Geometry check sheet. Reference: drawing and pictorial views, mm from the part's lowest x, y, z. A direction names the side the tool comes from. Round coordinates to 2 decimals unless told otherwise and drop trailing zeros. Write each loop counter-clockwise with the first axis right and the second up, starting at its lowest first coordinate (ties: lowest second). Pieces come first, ordered by that corner, then holes. Notation, with made-up numbers: (29.5, -8) -> (60.5, -8) arc R30 cw to (60.5, 26) -> close; hole circle Ø1 at (84, 34.5). An arc over 180 degrees is marked (long way). Write item = value, one per line.
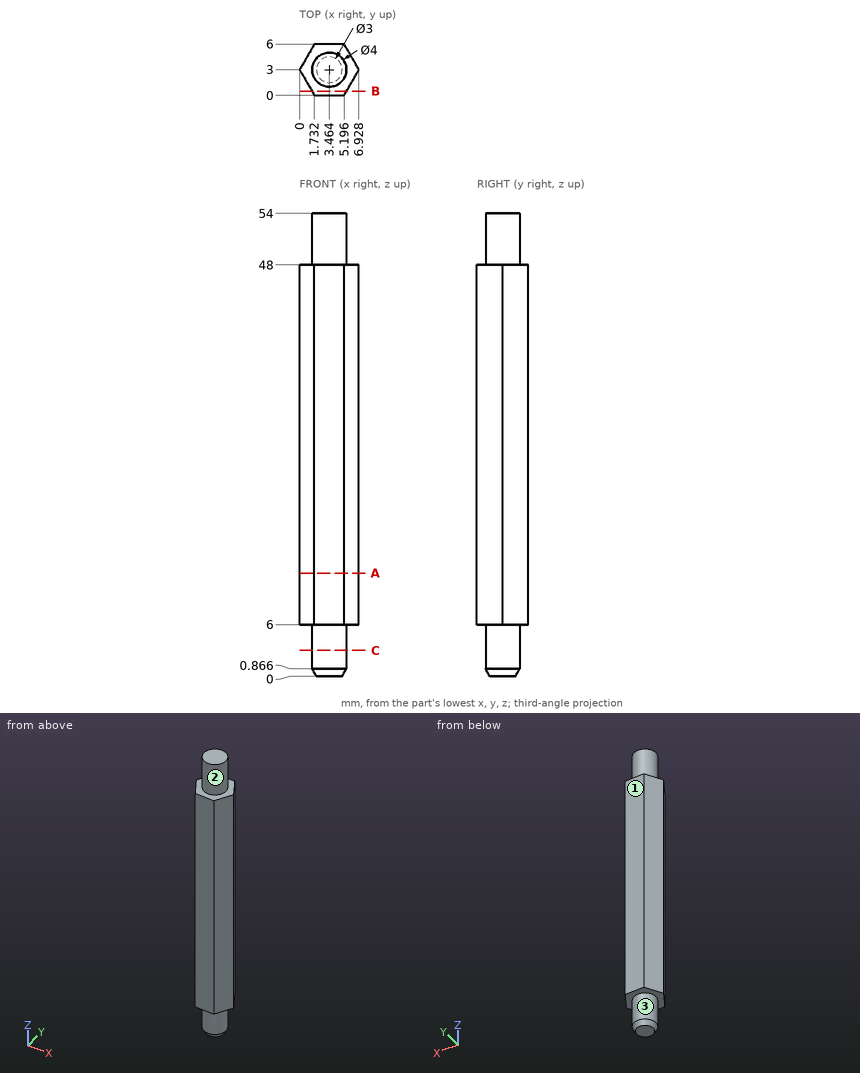
(1) Access from +Z, -Z, +X, -X, +Y, -Y to the whole of each face (thin tool, end or side, straight path). Record for the marked faces 1, 2 and 3.
Worked answers:
face_1 = +Z, -Z, +X, -X, +Y
face_2 = +Z
face_3 = -Z
(2) Sectioned sample at B-B on y = 0.5. Enter the section's corners in (x, z) (1 decimal).
Worked answers:
outline = (1.4, 6) -> (5.5, 6) -> (5.5, 48) -> (1.4, 48) -> close
(3) Go/stop test with a flat-tipped pin: P1, Ø2, axis at y = 4.5, z = 19.5, coming from the +X side. Record where the tip stops, or that it passes through.
Worked answers:
P1 = 6.64
(4) Material ranges on L1, parallel to Z at x = 2.75, y = 5.25; L2, parallel to Y at x = 5.75, z = 7.5; L3, parallel to Y at x = 6.25, z = 9 (1 decimal), recorded low to high. Write a range as [from, to].
Worked answers:
L1 = [6, 48]
L2 = [0.96, 5.04]
L3 = [1.8, 4.2]
(5) Sectioned sample at C-C on z = 3. Enter the section's corners in (x, y), then the cut area to 3 significant figures.
Worked answers:
outline = circle Ø4 at (3.46, 3)
area = 12.6 mm²
(6) Sectioned sample at A-A on z = 12. Enter the section's corners in (x, y), then the cut area to 3 significant figures.
Worked answers:
outline = (0, 3) -> (1.73, 0) -> (5.2, 0) -> (6.93, 3) -> (5.2, 6) -> (1.73, 6) -> close
area = 31.2 mm²
